Model file for the job. Use its own axes, mm. A direction names the side the tool comes from. Give positions to 0.01 mm unless a question says otherwise; leave off trailing zeros. Write each loop counter-clockwise with the first axis right and the second up, starting at its lowest first coordinate (ties: lowest second). Pieces come first, ordered by that corner, then holes.
```python
from build123d import *

# Parameters (mm, degrees)
F0_R     = 1.6
F1_DEPTH = 3


with BuildPart() as f1:
    # F0 (on Front) → F1 (new body)
    with BuildSketch(Plane.XZ):
        with BuildLine():
            add(Edge.make_bspline(
                [(0, 27.5), (-1.25, 24.166667), (-2.5, 20.833333), (-2.5, 17.5)],
                knots=[0, 0, 0, 0, 10.307764, 10.307764, 10.307764, 10.307764], degree=3))
            Line((0, 27.5), (0, 32.5))
            Line((0, 32.5), (0, 56.887164))
            ThreePointArc((0, 56.887164), (-5, 61.887164), (-10, 56.887164))
            Line((-10, 56.887164), (-10, 0))
            ThreePointArc((-10, 0), (-5, -5), (0, 0))
            Line((0, 0), (0, 7.5))
            add(Edge.make_bspline(
                [(-2.5, 17.5), (-2.5, 14.166667), (-1.25, 10.833333), (0, 7.5)],
                knots=[10.307764, 10.307764, 10.307764, 10.307764, 20.615528, 20.615528, 20.615528, 20.615528], degree=3))
        make_face()
        with Locations((-5, 0)):
            Circle(F0_R, mode=Mode.SUBTRACT)
        with BuildLine():
            Line((-6.25, 24.412836), (-6.25, 51.887164))
            ThreePointArc((-6.25, 51.887164), (-5, 53.137164), (-3.75, 51.887164))
            Line((-3.75, 51.887164), (-3.75, 24.412836))
            ThreePointArc((-3.75, 24.412836), (-5, 23.162836), (-6.25, 24.412836))
        make_face(mode=Mode.SUBTRACT)
    extrude(amount=F1_DEPTH)


solid = f1.part
```
1. Slice it at C-C, the plane y = -0.9. State how many separate pieces and enclosed holes the cut face has, and give its area (3 significant figures).
Calculated:
separate pieces: 1
enclosed holes: 2
area: 535 mm2
2. Slice it at B-B, the plane x = -5. Write the cut outline in (y, z), and give its area (3 significant figures).
Calculated:
outline: (-3, -5) - (0, -5) - (0, -1.6) - (-3, -1.6) - close; (-3, 1.6) - (0, 1.6) - (0, 23.16) - (-3, 23.16) - close; (-3, 53.14) - (0, 53.14) - (0, 61.89) - (-3, 61.89) - close
area: 101 mm2
3. Slice it at A-A, the plane z = 40. Write the cut outline in (x, y), and give its area (3 significant figures).
Calculated:
outline: (-10, -3) - (-6.25, -3) - (-6.25, 0) - (-10, 0) - close; (-3.75, -3) - (0, -3) - (0, 0) - (-3.75, 0) - close
area: 22.5 mm2
4. Which spindle directions (+Z, -Z, +X, -X, +Y, -Y) get a long thin tool onto all of the face, cutting with end or side? Do faces 4 (the flat face through (-7, -3, 29)), 5 (the cylindrical face through (-4.973, -1.479, 23.163)). Say none if no direction does.
Calculated:
face 4: +Z, -Z, +X, -X, -Y
face 5: +Y, -Y
5. Probe probe 1 along Z at (x, y) = (-5, -1.05); probe 2 along Z at (x, y) = (-5.5, -0.85); probe 3 along X at (y, z) = (-2.5, 52.5). List the from-to ranges inside material, lowest first.
Calculated:
probe 1: z = -5 to -1.6, 1.6 to 23.16, 53.14 to 61.89
probe 2: z = -4.97 to -1.52, 1.52 to 23.27, 53.03 to 61.86
probe 3: x = -10 to -6.09, -3.91 to 0
6. Slice it at D-D, the plane x = -9. Write the cut outline in (y, z).
Calculated:
outline: (-3, -3) - (0, -3) - (0, 59.89) - (-3, 59.89) - close
7. Pull direction Z, two halves, no side cores. Call faces 1 (the cylindrical face through (-6.6, -1.48, 0.07)), 2 (the cylindrical face through (-5, -1, -5)), 3 (the flat face through (0, -1, 4)): +Z half, -Z half, draft (parallel to the pull), parting line (faces both ways), or undercut.
Calculated:
face 1: undercut
face 2: -Z half
face 3: draft
